Can you work these out from the model? Positions are in its coordinate system, mm. Round coordinates to 2 decimals unless told otherwise and drop trailing zeros. Order: outer loops, then holes, each group sorted by start corner. A loop starts at its lowest first (then second) coordinate and runs counter-clockwise, first axis right, second up.
from build123d import *

# Parameters (mm, degrees)
BOSS_EXTRUDE1_DEPTH = 6
SCALE1_SCALE        = 0.75


with BuildPart() as part:
    # Sketch1 → Boss-Extrude1 (new body)
    with BuildSketch(Plane(origin=(0, 0, 0), x_dir=(1, 0, 0), z_dir=(0, 1, 0))):
        with BuildLine():
            Line((-10, 70), (-10, 90))
            Line((-10, 90), (-200, 90))
            Line((-200, 90), (-200, -120))
            Line((-200, -120), (300, -120))
            Line((300, -120), (300, -50))
            Line((300, -50), (110, -50))
            ThreePointArc((110, -50), (25.147186258, -14.852813742), (-10, 70))
        make_face()
    extrude(amount=-BOSS_EXTRUDE1_DEPTH)


with BuildPart() as part_1:
    # Scale1: scaled about (-15.320244378, -3, 38.872638603)
    add(part.part.scale(SCALE1_SCALE).moved(Location((-3.830061094, -0.75, 9.718159651))))


solid = part_1.part
(1) I'm going to push a flat-ended pin straight in: pin 1 Ø1 at (y, z) = (-4.5, -18.5) entering from +X. Where does the tip first touch, or does it pass through?
(2) I want a section at C-C, the plane z = -4. List the corners of the cut face in (x, y) for me.
(3) I want a section at A-A, the plane y = -3.3. List the corners of the cut face in (x, z) for me.
(4) I want a section at B-B, the plane x = 135. List the corners of the cut face in (y, z) for me, plus the area to 3 significant figures.
(5) If we mould it in two halves opening along Z, with no side actions, what happens to faces 1 (the face through (-11, -5.25, 37)), 2 (the face through (15.73, -2.97, 21.55))? For each: pulls with the +Z half, pulls with the -Z half, needs draft (parallel to the pull), parting line crosses it, or undercut.
(6) Please list where these lines run through material, in increasing order: probe 1 along Z at (x, y) = (78, -4.15); probe 2 along X at (y, z) = (-3.5, -6); probe 3 along X at (y, z) = (-3.45, -48.5).
Ans:
1. pin 1: stops at x = -7.85
2. outline: (-153.83, -5.25) - (-2.55, -5.25) - (-2.55, -0.75) - (-153.83, -0.75) - close
3. outline: (-153.83, -57.78) - (-11.33, -57.78) - (-11.33, -42.78) arc R90 cw to (78.67, 47.22) - (221.17, 47.22) - (221.17, 99.72) - (-153.83, 99.72) - close
4. outline: (-5.25, 47.22) - (-0.75, 47.22) - (-0.75, 99.72) - (-5.25, 99.72) - close
4. area: 236 mm2
5. face 1: needs draft
5. face 2: pulls with the -Z half
6. probe 1: z = 47.22 to 99.72
6. probe 2: x = -153.83 to -3.47
6. probe 3: x = -153.83 to -11.33
